Autodesk Inventor part; units mm, degrees
ref_plane "YZ Plane" through (0, 0, 0) normal (1, 0, 0) x (0, 1, 0)
ref_plane "XZ Plane" through (0, 0, 0) normal (0, 1, 0) x (-1, 0, 0)
ref_plane "XY Plane" through (0, 0, 0) normal (0, 0, 1) x (1, 0, 0)
sketch "Sketch1" plane through (0, 0, 0) normal (0, 1, 0) x (-1, 0, 0)
  line L0 (46.5, 30) -> (-46.5, 30)
  line L1 (-46.5, 30) -> (-46.5, -30)
  line L2 (-46.5, -30) -> (46.5, -30)
  line L3 (46.5, -30) -> (46.5, 30)
  line L4 (46.5, 30) -> (-46.5, -30) construction
  line L5 (-46.5, 30) -> (46.5, -30) construction
  circle A0 centre (-19.5, 0) radius 12.5
  line L6 (152.1746, 0) -> (-152.1746, 0) construction
  line L7 (0, 58.0523) -> (0, -58.0523) construction
  point P0 (0, 0)
  dimension "d0" = 93
  dimension "d2" = 25
  dimension "d4" = 60
  dimension "d5" = 27
extrude "Extrusion1" add sketch "Sketch1" along normal blind 5
sketch "Sketch2" plane through (0, 5, 0) normal (0, 1, 0) x (1, 0, 0)
  line L0 (-41.5, -25) -> (41.5, -25) construction
  line L1 (41.5, -25) -> (41.5, 25) construction
  line L2 (41.5, 25) -> (-41.5, 25) construction
  line L3 (-41.5, 25) -> (-41.5, -25) construction
  line L4 (-41.5, -25) -> (41.5, 25) construction
  line L5 (41.5, -25) -> (-41.5, 25) construction
  line L6 (46.5, 30) -> (-46.5, 30)
  line L7 (46.5, -30) -> (46.5, 30)
  point P0 (0, 0)
  dimension "d11" = 5
  dimension "d12" = 5
hole "Hole1" at (-41.5, 5, -25) at (41.5, 5, -25) at (41.5, 5, 25) at (-41.5, 5, 25) direction (0, -1, 0) diameter 3.4 end through all counterbore diameter 6.5 counterbore depth 3.4
sketch "Sketch3" plane through (0, 0, 0) normal (0, -1, 0) x (1, 0, 0)
  circle A0 centre (-41.5, 25) radius 3.25
  circle A1 centre (-41.5, 25) radius 4
  circle A2 centre (-41.5, 25) radius 1.7
  circle A3 centre (41.5, 25) radius 1.7
  circle A4 centre (41.5, -25) radius 1.7
  circle A5 centre (-41.5, -25) radius 1.7
  line L0 (46.5, 30) -> (46.5, -30)
  line L1 (-46.5, 30) -> (46.5, 30)
  line L2 (-46.5, -30) -> (-46.5, 30)
  line L3 (46.5, -30) -> (-46.5, -30)
  circle A6 centre (41.5, 25) radius 4
  circle A7 centre (-41.5, -25) radius 4
  circle A8 centre (41.5, -25) radius 4
  point P0 (0, 0)
  dimension "d22" = 83
  dimension "d25" = 50
  dimension "d28" = 8
extrude "Extrusion2" cut sketch "Sketch3" against normal blind 1 contours A0 | A1 | A2 | A3 | A4 | A5 | A6 | A7 | A8
sketch "Sketch4" plane through (0, 0, 0) normal (0, -1, 0) x (1, 0, 0)
  circle A0 centre (41.5, -25) radius 4
  circle A1 centre (-41.5, -25) radius 4
  circle A2 centre (41.5, 25) radius 4
  circle A3 centre (-41.5, 25) radius 4
  line L0 (46.5, 30) -> (46.5, -30)
  line L1 (-46.5, 30) -> (46.5, 30)
  line L2 (-46.5, -30) -> (-46.5, 30)
  line L3 (46.5, -30) -> (-46.5, -30)
  circle A4 centre (19.5, 0) radius 12.5
  circle A5 centre (19.5, 0) radius 14
  point P0 (0, 0)
  dimension "d31" = 28
extrude "Extrusion3" cut sketch "Sketch4" against normal through all contours A5
sketch "Sketch5" plane through (0, 0, 0) normal (0, -1, 0) x (1, 0, 0)
  line L0 (-35.5, 30) -> (-5.5, 30) construction
  line L1 (-5.5, 30) -> (-5.5, -30) construction
  line L2 (-5.5, -30) -> (-35.5, -30) construction
  line L3 (-35.5, -30) -> (-35.5, 30) construction
  line L4 (-65.1, 0) -> (65.1, 0)
  circle A0 centre (-30.5, 25) radius 4
  circle A1 centre (-10.5, 25) radius 4
  circle A2 centre (-30.5, -25) radius 4
  circle A3 centre (-10.5, -25) radius 4
  line L5 (-35.5, 30) -> (-5.5, -30) construction
  line L6 (-46.5, -30) -> (-46.5, 30)
  point P0 (0, 0)
  point P1 (-35.5, 0)
  point P2 (-20.5, 0)
  dimension "d34" = 60
  dimension "d35" = 30
  dimension "d36" = 8
  dimension "d37" = 5
  dimension "d38" = 5
  dimension "d41" = 20
  dimension "d44" = 50
  dimension "d47" = 26
extrude "Extrusion4" cut sketch "Sketch5" against normal blind 1
sketch "Sketch7" plane through (0, 5, 0) normal (0, 1, 0) x (1, 0, 0)
  circle A0 centre (-30.5, -25) radius 4 construction
  point P0 (0, 0)
hole "Hole2" at (-30.5, 5, 25) direction (0, -1, 0) diameter 3.4 end through all counterbore diameter 6.5 counterbore depth 3.4
pattern_linear "Rectangular Pattern1" count 2 spacing 50 along (0, 0, -1) count 2 spacing 20 along (1, 0, 0) of "Hole2"
sketch "Sketch8" plane through (0, 5, 0) normal (0, 1, 0) x (1, 0, 0)
  circle A0 centre (19.5, 0) radius 12.5
  circle A1 centre (19.5, 0) radius 21 construction
  line L0 (65.1, 0) -> (-65.1, 0)
  point P0 (0, 0)
  point P1 (-1.5, 0)
  point P2 (30, -18.1865)
  point P3 (30, 18.1865)
  dimension "d63" = 42
  dimension "d66" = 360
hole "Hole3" at (-1.5, 5, 0) at (30, 5, 18.1865) at (30, 5, -18.1865) direction (0, -1, 0) diameter 3.4 end through all
sketch "Sketch11" plane through (0, 0, 0) normal (0, -1, 0) x (1, 0, 0)
  circle A0 centre (19.5, 0) radius 14
  circle A1 centre (19.5, 0) radius 14.5
  circle A2 centre (19.5, 0) radius 14
  point P0 (0, 0)
  dimension "d81" = 0.5
extrude "Extrusion6" cut sketch "Sketch11" against normal blind 0.25
sketch "Sketch12" plane through (0, 5, 0) normal (0, 1, 0) x (1, 0, 0)
  circle A0 centre (19.5, 0) radius 14
  circle A1 centre (19.5, 0) radius 14.5
  point P0 (0, 0)
  dimension "d84" = 0.5
extrude "Extrusion7" cut sketch "Sketch12" against normal blind 0.25
properties part number "plate 2"
The model under review builds one solid part; all positions refer to its coordinate system, in mm. A direction names the side the tool comes from. Give positions to 0.01 mm unless a question says otherwise; leave off trailing zeros. Write each loop counter-clockwise with the first axis right and the second up, starting at its lowest first coordinate (ties: lowest second). Pieces come first, ordered by that corner, then holes.
1. Wall thickness on L1, parallel to Z at x = 41.5, y = 2.85; L2, parallel to X at y = 1.4, z = 25; L3, parallel to X at y = 3.3, z = -25: over which ranges is each line inside the solid? List them lowest first.
2. Add section A-A, the plane x = 41.5. Write out the cut boundary in (y, z).
3. Add section D-D, the plane x = 30. Write out the cut boundary in (y, z).
4. Add section B-B, the plane y = 3.1. Count the separate pieces of the cut face and the enclosed holes in it, plus the area to 3 significant figures.
5. Draft analysis for pull direction Z (two halves, no side actions). For faces 4 (the flat face through (-1, 2, 30)), 5 (the flat face through (1, 0, 0)), 6 (the cylindrical face through (31.51, 2.46, 18.97)), 7 (the cylindrical face through (-40, 1.3, 25.8)), state which applies: +Z half, -Z half, draft (parallel to the pull), parting line (faces both ways), or undercut.
6. For P1, Ø5.5, axis at x = 41.5, z = 25, coming from the -Y side; P2, Ø4.5, axis at x = -10.5, z = 25, coming from the +Y side, all flat-tipped, find the tip position at first contact; note any pin that passes through.
7. Tool access review of faces 1 (the cylindrical face through (-10.643, 3.276, -28.247)), 2 (the cylindrical face through (43, 1.3, -24.2)), 3 (the flat face through (-11, 1, -27)): name each direction out of +Z, -Z, +X, -X, +Y, -Y from which nothing blocks a thin tool from reaching the whole face with its end or side.
8. Add section C-C, the plane z = 8. Write out the cut boundary in (x, y), plus the area to 3 significant figures.
Worked answers:
1. L1: z = -30 to -28.25, -21.75 to 21.75, 28.25 to 30
1. L2: x = -46.5 to -43.2, -39.8 to -32.2, -28.8 to -12.2, -8.8 to 39.8, 43.2 to 46.5
1. L3: x = -46.5 to -44.75, -38.25 to -33.75, -27.25 to -13.75, -7.25 to 38.25, 44.75 to 46.5
2. outline: (0, -30) - (5, -30) - (5, -28.25) - (1.6, -28.25) - (1.6, -26.7) - (1, -26.7) - (1, -29) - (0, -29) - close; (0, -21) - (1, -21) - (1, -23.3) - (1.6, -23.3) - (1.6, -21.75) - (5, -21.75) - (5, 21.75) - (1.6, 21.75) - (1.6, 23.3) - (1, 23.3) - (1, 21) - (0, 21) - close; (0, 29) - (1, 29) - (1, 26.7) - (1.6, 26.7) - (1.6, 28.25) - (5, 28.25) - (5, 30) - (0, 30) - close
3. outline: (0, -30) - (5, -30) - (5, -19.89) - (0, -19.89) - close; (0, -16.49) - (5, -16.49) - (5, -10) - (4.75, -10) - (4.75, -9.26) - (0.25, -9.26) - (0.25, -10) - (0, -10) - close; (0, 10) - (0.25, 10) - (0.25, 9.26) - (4.75, 9.26) - (4.75, 10) - (5, 10) - (5, 16.49) - (0, 16.49) - close; (0, 19.89) - (5, 19.89) - (5, 30) - (0, 30) - close
4. separate pieces: 1
4. enclosed holes: 12
4. area: 4,670 mm2
5. face 4: +Z half
5. face 5: draft
5. face 6: undercut
5. face 7: undercut
6. P1: stops at y = 1
6. P2: stops at y = 1.6
7. face 1: +Y
7. face 2: +Y, -Y
7. face 3: -Y
8. outline: (-46.5, 0) - (7.41, 0) - (7.41, 0.25) - (8.01, 0.25) - (8.01, 4.75) - (7.41, 4.75) - (7.41, 5) - (-46.5, 5) - close; (30.99, 0.25) - (31.59, 0.25) - (31.59, 0) - (46.5, 0) - (46.5, 5) - (31.59, 5) - (31.59, 4.75) - (30.99, 4.75) - close
8. area: 350 mm2
